Could you check a few things on this model? Use its own coordinates, in mm. Give positions to 0.01 mm unless a question says otherwise; leave off trailing zeros. Write item = value, one per line.
from build123d import *

# Parameters (mm, degrees)
SKETCH1_RX              = 15.24
SKETCH1_RY              = 9.525
BOSS_EXTRUDE2_DEPTH     = 34.29
CUT_EXTRUDE1_START      = -0.635
SKETCH3_RX              = 14.605
SKETCH3_RY              = 8.89
CUT_EXTRUDE1_DEPTH      = 33.02
CUT_EXTRUDE3_START      = -0.635
CUT_EXTRUDE3_DEPTH      = 32.7025
SKETCH6_W               = 32.06646649
SKETCH6_H               = 9.119465297
CUT_EXTRUDE4_DEPTH      = 40.3225
CUT_EXTRUDE4_DEPTH_BACK = 32.7025
SKETCH7_W               = 29.517013218
SKETCH7_H               = 33.655
CUT_EXTRUDE5_DEPTH      = 1.93413
SKETCH8_W               = 0.327986782
SKETCH8_H               = 0.3175
CUT_EXTRUDE6_DEPTH      = 1.93413
SKETCH9_W               = 0.327986782
SKETCH9_H               = 0.635
CUT_EXTRUDE7_DEPTH      = 1.93413


with BuildPart() as part:
    # Sketch1 → Boss-Extrude2 (new body)
    with BuildSketch(Plane.XY):
        with Locations(Location((0, 0), (0, 0, 180))):
            Ellipse(SKETCH1_RX, SKETCH1_RY)
    extrude(amount=BOSS_EXTRUDE2_DEPTH)

    # Sketch3 → Cut-Extrude1 (cut)
    with BuildSketch(Plane.XY.offset(34.29).offset(CUT_EXTRUDE1_START)):
        with Locations(Location((0, 0), (0, 0, 4.189e-06))):
            Ellipse(SKETCH3_RX, SKETCH3_RY)
    extrude(amount=-CUT_EXTRUDE1_DEPTH, mode=Mode.SUBTRACT)

    # Sketch4 → Cut-Extrude3 (cut)
    with BuildSketch(Plane.XY.offset(34.29).offset(CUT_EXTRUDE3_START)):
        with BuildLine():
            Line((-14.9225, 0), (0, 0))
            Line((0, 0), (0, 9.525))
            add(Edge.make_bspline(
                [(0, 9.525), (-12.403805408, 9.525), (-14.9225, 1.934129503)],
                knots=[4.71238898, 4.71238898, 4.71238898, 6.078705108, 6.078705108, 6.078705108], degree=2, weights=[1, 0.775583076, 1]))
            Line((-14.9225, 1.934129503), (-14.9225, 0))
        make_face()
        with BuildLine():
            Line((0, 0), (14.9225, 0))
            Line((14.9225, 0), (14.9225, 1.934129503))
            add(Edge.make_bspline(
                [(14.9225, 1.934129503), (12.403805408, 9.525), (0, 9.525)],
                knots=[3.346072853, 3.346072853, 3.346072853, 4.71238898, 4.71238898, 4.71238898], degree=2, weights=[1, 0.775583076, 1]))
            Line((0, 9.525), (0, 0))
        make_face()
    extrude(amount=-CUT_EXTRUDE3_DEPTH, mode=Mode.SUBTRACT)

    # Sketch6 → Cut-Extrude4 (cut, two sides)
    with BuildSketch(Plane(origin=(0, 0, 33.655), x_dir=(-1, 0, 0), z_dir=(0, 0, -1))) as cut_extrude4_sk:
        with Locations((1.110733245, 6.493862152)):
            Rectangle(SKETCH6_W, SKETCH6_H)
    extrude(amount=CUT_EXTRUDE4_DEPTH, mode=Mode.SUBTRACT)
    extrude(cut_extrude4_sk.sketch, amount=-CUT_EXTRUDE4_DEPTH_BACK, mode=Mode.SUBTRACT)

    # Sketch7 → Cut-Extrude5 (cut)
    with BuildSketch(Plane(origin=(0, 1.934129503, 0), x_dir=(1, 0, 0), z_dir=(0, 1, 0))):
        with Locations((0.163993391, -17.145)):
            Rectangle(SKETCH7_W, SKETCH7_H)
    extrude(amount=-CUT_EXTRUDE5_DEPTH, mode=Mode.SUBTRACT)

    # Sketch8 → Cut-Extrude6 (cut)
    with BuildSketch(Plane(origin=(0, 1.934129503, 0), x_dir=(1, 0, 0), z_dir=(0, 1, 0))):
        with Locations((-14.758506609, -33.81375)):
            Rectangle(SKETCH8_W, SKETCH8_H)
    extrude(amount=-CUT_EXTRUDE6_DEPTH, mode=Mode.SUBTRACT)

    # Sketch9 → Cut-Extrude7 (cut)
    with BuildSketch(Plane(origin=(0, 1.934129503, 0), x_dir=(1, 0, 0), z_dir=(0, 1, 0))):
        with Locations((-14.758506609, -0.635)):
            Rectangle(SKETCH9_W, SKETCH9_H)
    extrude(amount=-CUT_EXTRUDE7_DEPTH, mode=Mode.SUBTRACT)


solid = part.part
1. Thinking about a two-plate mould opening in Z: for faces 1 (the face through (0, -3, 0)), 2 (the face through (0, -3, 34.29)), 3 (the face through (0, -3, 33.655)), which applies, pulls with the +Z half, pulls with the -Z half, needs draft (parallel to the pull), parting line crosses it, or undercut?
Filled sheet:
face_1 = pulls with the -Z half
face_2 = pulls with the +Z half
face_3 = undercut
2. I need wall thicknesses on line 1 (Z direction, x = -4, y = -1) (3 decimals); line 2 (X direction, y = -0.5, z = 27.5); line 3 (X direction, y = 0.75, z = 17). Which ranges of each line are inside material? Lowest first, please.
Filled sheet:
line_1 = 0 to 0.635, 33.655 to 34.29
line_2 = -15.22 to -14.58, 14.58 to 15.22
line_3 = -15.19 to -14.92, 14.92 to 15.19
3. For pin 1 (1 mm diameter, centred on y = 1, z = 22.5, fed in from -X); pin 2 (0.6 mm diameter, centred on y = 1, z = 23, fed in from +X); pin 3 (9 mm diameter, centred on x = 3, z = 18.5, fed in from +Y), each with a flat end and sliding along its axis, tell me the tip position at first contact or that it passes through.
Filled sheet:
pin_1 = -15.22
pin_2 = 15.2
pin_3 = -7.63
